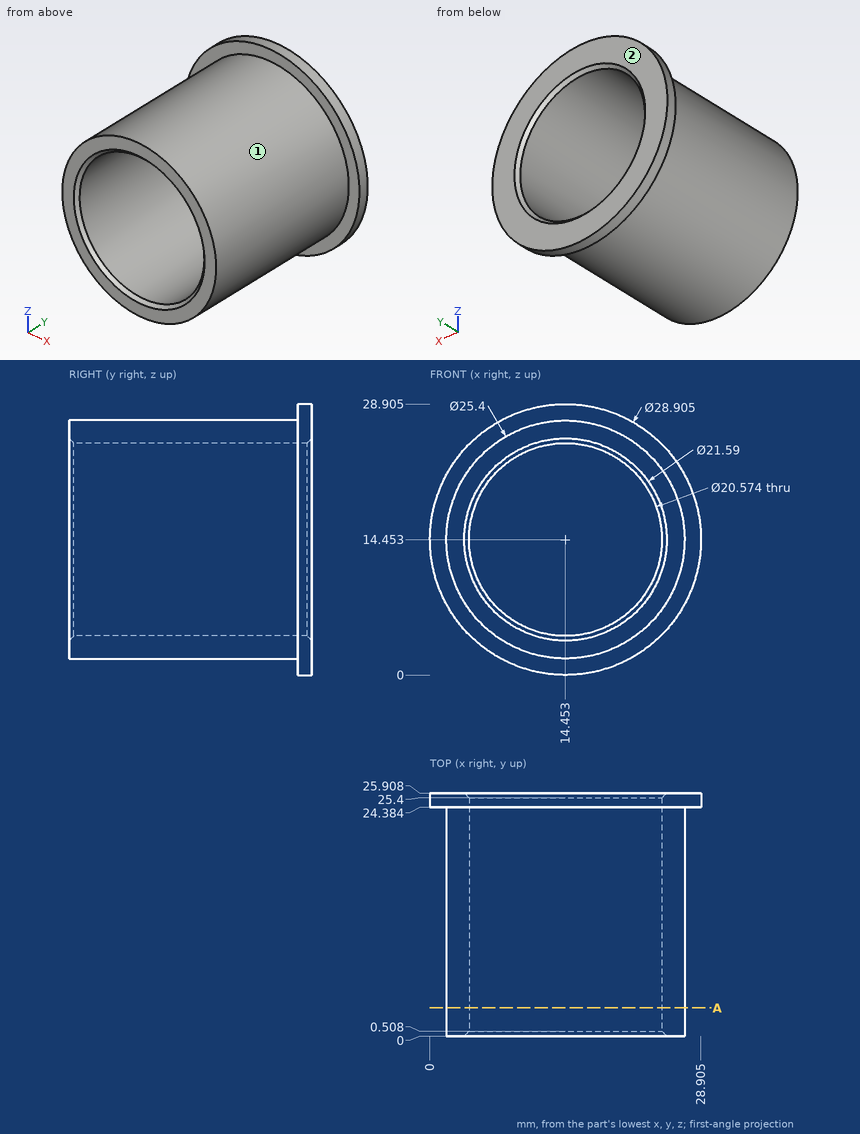
Input: dimensioned drawing with shaded views. Units: mm. Origin: part minimum x, y, z. A direction names the side the tool comes from. Give positions to 0.01 mm unless a question says otherwise; leave off trailing zeros. Write each loop counter-clockwise with the first axis right and the second up, starting at its lowest first coordinate (ties: lowest second). Pieces come first, ordered by that corner, then holes. Notation, with made-up numbers: (-21.75, 81) -> (6.25, 81) arc R37 ccw to (6.25, 118) -> close; hole circle Ø4 at (21, 48.25). An arc over 180 degrees is marked (long way). Return JSON: item names as keys, results as strings. Group by question number.
1. Section A-A, the plane y = 3. Output: boundary loops of the cut face in (x, z) (1 decimal), then the cut area to 3 significant figures.
2. Access query for the marked faces 1 and 2. Directions: +Z, -Z, +X, -X, +Y, -Y. A direction counts if a zero-diameter tool reaches every point of the face in a straight line with its end or side. Return the directions, or none.
3. Material intervals for line 1 (Z direction, x = 14.25, y = 7.25) (1 decimal); line 2 (X direction, y = 15, z = 14) (1 decimal); line 3 (Y direction, x = 24, z = 5.25), sorted ascending. Write a range as from..to.
4. Pin query (flat end, axial travel): pin 1 Ø3 at (x, y) = (24.5, 21.5) entering from +Z (1 decimal); pin 2 Ø8 at (x, y) = (25, 15.5) entering from +Z (1 decimal); pin 3 Ø3 at (y, z) = (18, 9.5) entering from +X (1 decimal). Return the tip coordinate at first contact, or that it passes through.
Determined:
{
 "1": {"outline": "circle Ø25.4 at (14.5, 14.5); hole circle Ø20.6 at (14.5, 14.5)", "area": "174 mm2"},
 "2": {"face 1": "-Y", "face 2": "+Z, -Z, +X, -X, +Y"},
 "3": {"line 1": "z = 1.8..4.2, 24.7..27.2", "line 2": "x = 1.8..4.2, 24.7..27.1", "line 3": "y = 24.38..25.91"},
 "4": {"pin 1": "stops at z = 23.8", "pin 2": "stops at z = 25.3", "pin 3": "stops at x = 26.7"}
}
